Work out the finished part from the listing and answer in its coordinate system (mm). Round coordinates to 2 decimals unless told otherwise and drop trailing zeros. Write each loop counter-clockwise with the first axis right and the second up, starting at its lowest first coordinate (ties: lowest second). Pieces come first, ordered by that corner, then holes.
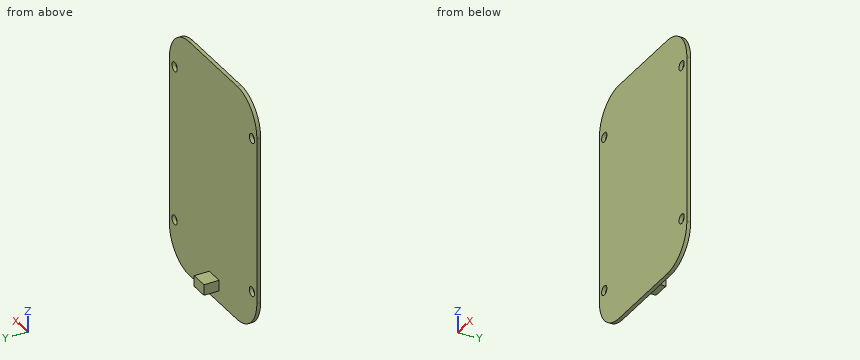
from build123d import *

# Parameters (mm, degrees)
BOSS_EXTRUDE1_DEPTH = 1.3
SKETCH2_R           = 1.6
CUT_EXTRUDE1_DEPTH  = 1.3
SKETCH3_W           = 6
SKETCH3_H           = 3.7
BOSS_EXTRUDE2_DEPTH = 5.2


with BuildPart() as part:
    # Sketch1 → Boss-Extrude1 (new body)
    with BuildSketch(Plane(origin=(0, 0, 0), x_dir=(1, 0, 0), z_dir=(0, 1, 0))):
        with BuildLine():
            Line((-20.801575534, 33.774503622), (8.728424466, 33.774503622))
            ThreePointArc((8.728424466, 33.774503622), (17.21370584, 30.259784996), (20.728424466, 21.774503622))
            Line((20.728424466, 21.774503622), (20.728424466, -35.625496378))
            ThreePointArc((20.728424466, -35.625496378), (17.21370584, -44.110777752), (8.728424466, -47.625496378))
            Line((8.728424466, -47.625496378), (-20.801575534, -47.625496378))
            ThreePointArc((-20.801575534, -47.625496378), (-29.286856908, -44.110777752), (-32.801575534, -35.625496378))
            Line((-32.801575534, -35.625496378), (-32.801575534, 21.774503622))
            ThreePointArc((-32.801575534, 21.774503622), (-29.286856908, 30.259784996), (-20.801575534, 33.774503622))
        make_face()
    extrude(amount=BOSS_EXTRUDE1_DEPTH)

    # Sketch2 → Cut-Extrude1 (cut)
    with BuildSketch(Plane(origin=(0, 1.3, 0), x_dir=(1, 0, 0), z_dir=(0, 1, 0))):
        with Locations(Location((-29.801575534, 19.274503622, 0), (0, 0, 270))):
            Circle(SKETCH2_R)
        with Locations(Location((17.518424466, 19.274503622, 0), (0, 0, 270))):
            Circle(SKETCH2_R)
        with Locations(Location((17.518424466, -34.195496378, 0), (0, 0, 270))):
            Circle(SKETCH2_R)
        with Locations(Location((-29.801575534, -34.195496378, 0), (0, 0, 270))):
            Circle(SKETCH2_R)
    extrude(amount=-CUT_EXTRUDE1_DEPTH, mode=Mode.SUBTRACT)

    # Sketch3 → Boss-Extrude2 (add)
    with BuildSketch(Plane(origin=(0, 1.3, 0), x_dir=(1, 0, 0), z_dir=(0, 1, 0))):
        with Locations((-6.731575534, 27.794503622)):
            Rectangle(SKETCH3_W, SKETCH3_H)
    extrude(amount=BOSS_EXTRUDE2_DEPTH)


solid = part.part
Q1. Find the intervals of material crossed by L1, parallel to Y at x = 5.5, z = 3; L2, parallel to Z at x = -4, y = 6; L3, parallel to X at y = 1, z = -27, in increasing order.
Q2. Find section A-A (x = -6). Determine the outline of the cut face in (y, z), plus the area to 3 significant figures.
Q3. Find section B-B (y = 2.25). Determine the outline of the cut face in (x, z).
Q4. Find section C-C (z = -27.5). Determine the outline of the cut face in (x, y).
Q5. Given pin 1 (3 mm diameter, centred on y = 3.5, z = -27.5, fed in from +X); pin 2 (4 mm diameter, centred on x = 17.52, z = 34.2, fed in from +Y); pin 3 (2.5 mm diameter, centred on x = -5.5, y = 3.5, fed in from -Z), each flat-ended and moving along its own axis, determine where each tip first touches the part or whether it passes through.
Q6. Find section D-D (z = -3). Determine the outline of the cut face in (x, y), plus the area to 3 significant figures.
Report:
1. L1: y = 0 to 1.3
1. L2: z = -29.64 to -25.94
1. L3: x = -31.6 to 19.53
2. outline: (0, -33.77) - (1.3, -33.77) - (1.3, -29.64) - (6.5, -29.64) - (6.5, -25.94) - (1.3, -25.94) - (1.3, 47.63) - (0, 47.63) - close
2. area: 125 mm2
3. outline: (-9.73, -29.64) - (-3.73, -29.64) - (-3.73, -25.94) - (-9.73, -25.94) - close
4. outline: (-31.35, 0) - (19.27, 0) - (19.27, 1.3) - (-3.73, 1.3) - (-3.73, 6.5) - (-9.73, 6.5) - (-9.73, 1.3) - (-31.35, 1.3) - close
5. pin 1: stops at x = -3.73
5. pin 2: stops at y = 1.3
5. pin 3: stops at z = -29.64
6. outline: (-32.8, 0) - (20.73, 0) - (20.73, 1.3) - (-32.8, 1.3) - close
6. area: 69.6 mm2
